from build123d import *

# Parameters (mm, degrees)
F0_R     = 9.92251
F0_W     = 76.2
F0_H     = 7.9375
F1_DEPTH = 88.9
F2_R     = 10.3251
F3_DEPTH = 7.9385
F5_DEPTH = 133.351


with BuildPart() as f1:
    # F0 (on Front) → F1 (new body)
    with BuildSketch(Plane.XZ):
        with BuildLine():
            Line((0, 44.45), (0, 0))
            Line((0, 0), (57.15, 0))
            Line((57.15, 0), (57.15, 7.9375))
            Line((57.15, 7.9375), (57.15, 44.45))
            ThreePointArc((57.15, 44.45), (28.575, 73.025), (0, 44.45))
        make_face()
        with Locations((28.575, 44.45)):
            Circle(F0_R, mode=Mode.SUBTRACT)
        with Locations((95.25, 3.96875)):
            Rectangle(F0_W, F0_H)
    extrude(amount=F1_DEPTH)

    # F2 (on face) → F3 (cut, through all)
    with BuildSketch(Plane.XY.offset(7.9375)):
        with Locations((73.025, -44.45)):
            Circle(F2_R)
        with Locations((111.125, -44.45)):
            Circle(F2_R)
        with BuildLine():
            Line((133.35, 0), (57.15, 0))
            Line((57.15, 0), (57.15, -15.875))
            ThreePointArc((57.15, -15.875), (59.009872, -20.365128), (63.5, -22.225))
            Line((63.5, -22.225), (111.125, -22.225))
            ThreePointArc((111.125, -22.225), (126.840448, -28.734552), (133.35, -44.45))
            Line((133.35, -44.45), (133.35, 0))
        make_face()
        with BuildLine():
            Line((133.35, -88.9), (133.35, -44.45))
            ThreePointArc((133.35, -44.45), (126.840448, -60.165448), (111.125, -66.675))
            Line((111.125, -66.675), (63.5, -66.675))
            ThreePointArc((63.5, -66.675), (59.009872, -68.534872), (57.15, -73.025))
            Line((57.15, -73.025), (57.15, -88.9))
            Line((57.15, -88.9), (133.35, -88.9))
        make_face()
    extrude(amount=-F3_DEPTH, mode=Mode.SUBTRACT)

    # F4 (on Right) → F5 (cut, through all)
    with BuildSketch(Plane.YZ):
        with BuildLine():
            Line((-7.9375, 73.025), (-80.9625, 73.025))
            Line((-80.9625, 73.025), (-80.9625, 12.7))
            ThreePointArc((-80.9625, 12.7), (-79.567596, 9.332404), (-76.2, 7.9375))
            Line((-76.2, 7.9375), (-12.7, 7.9375))
            ThreePointArc((-12.7, 7.9375), (-9.332404, 9.332404), (-7.9375, 12.7))
            Line((-7.9375, 12.7), (-7.9375, 73.025))
        make_face()
        with BuildLine():
            ThreePointArc((-76.2, 0), (-85.180256, 3.719744), (-88.9, 12.7))
            Line((-88.9, 12.7), (-88.9, 0))
            Line((-88.9, 0), (-76.2, 0))
        make_face()
        with BuildLine():
            Line((-12.7, 0), (0, 0))
            Line((0, 0), (0, 12.7))
            ThreePointArc((0, 12.7), (-3.719744, 3.719744), (-12.7, 0))
        make_face()
    extrude(amount=F5_DEPTH, mode=Mode.SUBTRACT)


solid = f1.part
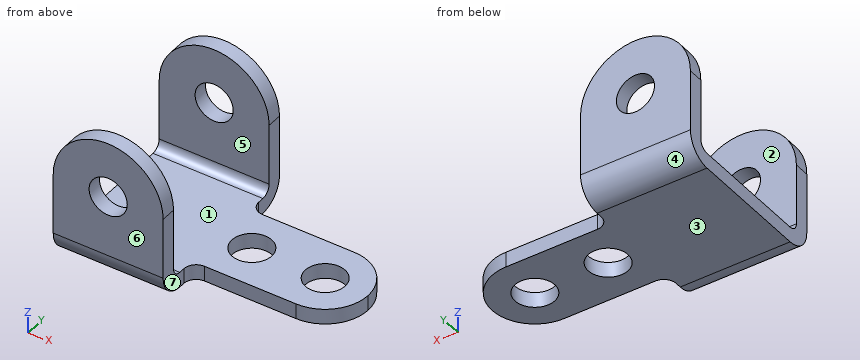
Source: CAD feature listing. Evaluate the final solid. Frame: model axes, mm. Face numbers are marked on the shaded views. A direction names the side the tool comes from. Round coordinates to 2 decimals unless told otherwise and drop trailing zeros. Loops run counter-clockwise (first coordinate to the right, second up) from the corner with the lowest first, then second, coordinate; pieces in that order, holes last.
Q1. Access query for the marked faces 5, 6 and 7. Directions: +Z, -Z, +X, -X, +Y, -Y. A direction counts if a zero-diameter tool reaches every point of the face in a straight line with its end or side. Return the directions, or none.
Q2. Section A-A, the plane z = 15.5. Return loops of the section in (x, y), plus the area to 3 significant figures.
Q3. Section C-C, the plane x = 11. Return loops of the section in (y, z) (1 decimal), plus the area to 3 significant figures.
Q4. Section D-D, the plane y = -70.5. Return loops of the section in (x, z), plus the area to 3 significant figures.
Q5. First-contact query: P1, Ø12, axis at x = 65.5, z = 12.5, coming from the +Y side; P2, Ø17.5, axis at y = -8.5, z = 31.5, coming from the +X side; P3, Ø10, axis at x = 22.5, y = -77.5, coming from the +Z side. Flat tips, straight axial feed; report the tip coordinate or a pass-through.
Q6. Ray query, line 1 (X direction, y = -44, z = 3); line 2 (Y direction, x = 28, z = 19); line 3 (Z direction, x = 20.5, y = -23.5). Return the intervals inside material, ascending.
Q7. Mould query, pull axis Y, two halves, no side actions, for the marked faces 1, 2, 3 and 4. Classes: pulls with the +Y half, pulls with the -Y half, needs draft (parallel to the pull), parting line crosses it, or undercut.
Q8. Section B-B, the plane y = -51. Return loops of the section in (x, z).
Solutions:
1. face 5: +Z, +X, -X
1. face 6: +Z, -Z, +X, -X, -Y
1. face 7: +Z, -Z, +X, -Y
2. outline: (0, -88.9) - (57.15, -88.9) - (57.15, -80.96) - (0, -80.96) - close; (0, -7.94) - (57.15, -7.94) - (57.15, 0) - (0, 0) - close
2. area: 907 mm2
3. outline: (-88.9, 12.7) arc R12.7 ccw to (-76.2, 0) - (-12.7, 0) arc R12.7 ccw to (0, 12.7) - (0, 67) - (-7.9, 67) - (-7.9, 12.7) arc R4.8 cw to (-12.7, 7.9) - (-76.2, 7.9) arc R4.8 cw to (-81, 12.7) - (-81, 67) - (-88.9, 67) - close
3. area: 1,580 mm2
4. outline: (0, 0) - (57.67, 0) - (57.67, 7.94) - (0, 7.94) - close
4. area: 458 mm2
5. P1: stops at y = -21.94
5. P2: stops at x = 57.15
5. P3: stops at z = 72.92
6. line 1: x = 0 to 62.71, 83.34 to 100.81, 121.44 to 133.35
6. line 2: y = -88.9 to -80.96, -7.94 to 0
6. line 3: z = 0 to 7.94
7. face 1: undercut
7. face 2: undercut
7. face 3: needs draft
7. face 4: pulls with the +Y half
8. outline: (0, 0) - (65.04, 0) - (65.04, 7.94) - (0, 7.94) - close; (81.01, 0) - (103.14, 0) - (103.14, 7.94) - (81.01, 7.94) - close; (119.11, 0) - (132.36, 0) - (132.36, 7.94) - (119.11, 7.94) - close
